Can you work these out from the model? Positions are in its coordinate system, mm. Face numbers are marked on the shaded views. A direction names the side the tool comes from. Coordinates: 2 decimals unless noted, no trailing zeros. Loops run counter-clockwise (first coordinate to the right, second up) from the corner with the lowest first, then second, coordinate; pieces in that order, holes last.
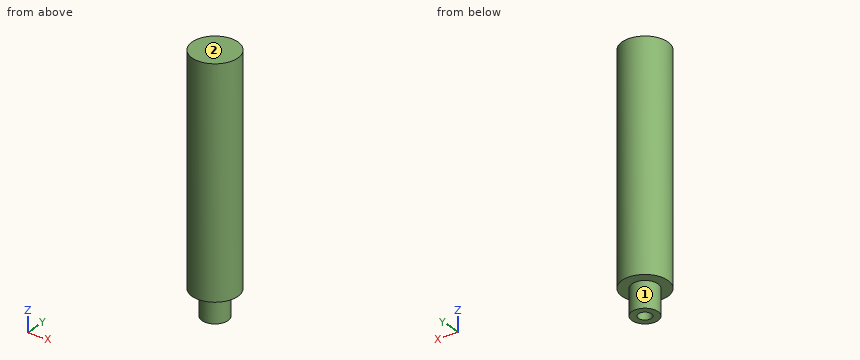
```python
from build123d import *

# Parameters (mm, degrees)
F0_R     = 13.97
F1_DEPTH = 152.4
F2_R     = 13.97
F2_R_2   = 7.9375
F3_DEPTH = 15.875
F4_R     = 3.96875
F5_DEPTH = 127


with BuildPart() as f1:
    # F0 (on Top) → F1 (new body)
    with BuildSketch(Plane.XY):
        Circle(F0_R)
    extrude(amount=F1_DEPTH)

    # F2 (on face) → F3 (cut)
    with BuildSketch(Plane(origin=(0, 0, 0), x_dir=(1, 0, 0), z_dir=(0, 0, -1))):
        Circle(F2_R)
        Circle(F2_R_2, mode=Mode.SUBTRACT)
    extrude(amount=-F3_DEPTH, mode=Mode.SUBTRACT)

    # F4 (on face) → F5 (cut)
    with BuildSketch(Plane(origin=(0, 0, 0), x_dir=(1, 0, 0), z_dir=(0, 0, -1))):
        Circle(F4_R)
    extrude(amount=-F5_DEPTH, mode=Mode.SUBTRACT)


solid = f1.part
```
Item 1: I need wall thicknesses on line 1 along X through (y, z) = (0, 101.5); line 2 along X through (y, z) = (-3, 39). Which ranges of each line are inside material? Lowest first, please.
Results are:
line 1: x = -13.97 to -3.97, 3.97 to 13.97
line 2: x = -13.64 to -2.6, 2.6 to 13.64
Item 2: On a 3-axis mill with a long thin cutter (end or side, diameter ignored), from which of +Z, -Z, +X, -X, +Y, -Y can I reach the whole of each face in a straight line? I mean the marked faces 1 and 2. Say none if no direction works.
Results are:
face 1: -Z
face 2: +Z, +X, -X, +Y, -Y
Item 3: Suppose I cut it at D-D, the plane y = -6. Please give me the cut outline in (x, z) (3 decimals), plus the area to 3 significant figures.
Results are:
outline: (-12.616, 15.875) - (-5.197, 15.875) - (-5.197, 0) - (5.197, 0) - (5.197, 15.875) - (12.616, 15.875) - (12.616, 152.4) - (-12.616, 152.4) - close
area: 3,610 mm2
Item 4: Suppose I cut it at A-A, the plane x = 0. Please give me the cut outline in (y, z) (1 decimal), plus the area to 3 significant figures.
Results are:
outline: (-14, 15.9) - (-7.9, 15.9) - (-7.9, 0) - (-4, 0) - (-4, 127) - (4, 127) - (4, 0) - (7.9, 0) - (7.9, 15.9) - (14, 15.9) - (14, 152.4) - (-14, 152.4) - close
area: 3,060 mm2
Item 5: Suppose I cut it at C-C, the plane z = 31. Please give me the cut outline in (x, y), plus the area to 3 significant figures.
Results are:
outline: circle Ø27.94 at (0, 0); hole circle Ø7.94 at (0, 0)
area: 564 mm2
Item 6: I'm going to push flat-ended pins straight in: P1, Ø12, axis at y = -6.5, z = 80, coming from the -X side; P2, Ø2.5, axis at x = 1, y = 1, coming from the -Z side; P3, Ø10, axis at x = 10.5, z = 60.5, coming from the +Y side. Where does each tip first touch, or does it pass through?
Results are:
P1: stops at x = -13.96
P2: stops at z = 127
P3: stops at y = 12.84
